```python
from build123d import *

# Parameters (mm, degrees)
F0_W     = 95
F0_H     = 13
F1_DEPTH = 11
F2_W     = 90.2
F2_H     = 8.4
F3_DEPTH = 7
F4_R     = 1.75
F5_DEPTH = 4


# Not quite as in the source:
# - a pattern or mirror of a feature is missing from the dataset's text; its kind, count and spacing are read off the source's solid


with BuildPart() as f1:
    # F0 (on Front) → F1 (new body)
    with BuildSketch(Plane.XZ):
        Rectangle(F0_W, F0_H)
    extrude(amount=F1_DEPTH)

    # F2 (on face) → F3 (cut)
    with BuildSketch(Plane.XZ.offset(11)):
        Rectangle(F2_W, F2_H)
    extrude(amount=-F3_DEPTH, mode=Mode.SUBTRACT)

    # F4 (on face) → F5 (cut, through all)
    with BuildSketch(Plane.XZ.offset(4)):
        with Locations((-30, 0)):
            Circle(F4_R)
    f5 = extrude(amount=-F5_DEPTH, mode=Mode.SUBTRACT)

    # F5_copies: F5 across plane
    add(f5.mirror(Plane(origin=(0, 0, 0), x_dir=(0, 0, 1), z_dir=(1, 0, 0))), mode=Mode.SUBTRACT)


solid = f1.part
```
Verification items for the finished model (mm, model axes). A direction names the side the tool comes from. Round coordinates to 2 decimals unless told otherwise and drop trailing zeros. Write each loop counter-clockwise with the first axis right and the second up, starting at its lowest first coordinate (ties: lowest second). Pieces come first, ordered by that corner, then holes.
1. Access from +Z, -Z, +X, -X, +Y, -Y to the whole of each face (thin tool, end or side, straight path). Record for faces 5 (the flat face through (-0.7, -11, 4.4)), 6 (the flat face through (-45.1, -8, 0)).
2. Draft check along X on faces 1 (the flat face through (-1, -5, -6.5)), 2 (the flat face through (47.5, -5, 0)), 3 (the flat face through (45.1, -8, 0)), 4 (the cylindrical face through (31.75, -2.03, 0.08)). Enter one of: +X half, -X half, draft (parallel to the pull), parting line (faces both ways), or undercut.
3. Gauge pin test, flat ends, axial feed: P1, Ø2, axis at x = 7.5, z = 2, coming from the -Y side; P2, Ø5.5, axis at x = -30, z = 0, coming from the +Y side. Record the tip position at first contact, or that the pin passes through.
4. Section check D-D on y = -1.25. Enter the section's corners in (x, z).
5. Section check B-B on z = 0. Enter the section's corners in (x, y).
6. Section check A-A on x = 30. Enter the section's corners in (y, z).
7. Section check C-C on y = -5. Enter the section's corners in (x, z), plus the area to 3 significant figures.
8. Scan lines: L1, parallel to X at y = -10.5, z = 2.5; L2, parallel to Z at x = 1, y = -6.25; L3, parallel to Z at x = -30, y = -1.2. Record each from-to range of solid material in increasing order.
Answer:
1. face 5: +Z, -Z, +X, -X, -Y
1. face 6: -Y
2. face 1: draft
2. face 2: +X half
2. face 3: undercut
2. face 4: undercut
3. P1: stops at y = -4
3. P2: stops at y = 0
4. outline: (-47.5, -6.5) - (47.5, -6.5) - (47.5, 6.5) - (-47.5, 6.5) - close; hole circle Ø3.5 at (-30, 0); hole circle Ø3.5 at (30, 0)
5. outline: (-47.5, -11) - (-45.1, -11) - (-45.1, -4) - (-31.75, -4) - (-31.75, 0) - (-47.5, 0) - close; (-28.25, -4) - (28.25, -4) - (28.25, 0) - (-28.25, 0) - close; (31.75, -4) - (45.1, -4) - (45.1, -11) - (47.5, -11) - (47.5, 0) - (31.75, 0) - close
6. outline: (-11, -6.5) - (0, -6.5) - (0, -1.75) - (-4, -1.75) - (-4, -4.2) - (-11, -4.2) - close; (-11, 4.2) - (-4, 4.2) - (-4, 1.75) - (0, 1.75) - (0, 6.5) - (-11, 6.5) - close
7. outline: (-47.5, -6.5) - (47.5, -6.5) - (47.5, 6.5) - (-47.5, 6.5) - close; hole (-45.1, -4.2) - (45.1, -4.2) - (45.1, 4.2) - (-45.1, 4.2) - close
7. area: 477 mm2
8. L1: x = -47.5 to -45.1, 45.1 to 47.5
8. L2: z = -6.5 to -4.2, 4.2 to 6.5
8. L3: z = -6.5 to -1.75, 1.75 to 6.5
